Input: part model. Units: mm. Frame: model coordinates. Face numbers are marked on the shaded views. A direction names the side the tool comes from. Coordinates: 2 decimals unless noted, no trailing zeros. Write each loop counter-clockwise with the first axis right and the second up, starting at its lowest first coordinate (ties: lowest second). Pieces come first, ordered by that corner, then holes. Notation, with made-up numbers: (14, -9.75) - (60, -9.75) arc R37 ccw to (60, 26.25) - close; hole circle Ø6 at (9.25, 29). An arc over 180 degrees is marked (long way). Use a Markdown table: item, result. Add a question column.
Q1. Section query D-D (z = 0). Return the cut outline in (x, y).
Q2. Section query C-C (y = 0.7). Return the cut outline in (x, z), then the cut area to 3 significant figures.
Q3. Set-up query: the marked faces 5 and 6. Return all of +Z, -Z, +X, -X, +Y, -Y with unobstructed straight access to the full face (end or side cutting, diameter ignored); none if empty.
Q4. Section query A-A (x = -7.5). Return the cut outline in (y, z).
Q5. Section query B-B (x = 7.5). Return the cut outline in (y, z), then the cut area to 3 significant figures.
Q6. Pin query (flat end, axial travel): P1, Ø1.8, axis at y = 2, z = 0.5, coming from the +X side; P2, Ø6, axis at x = 0, z = 0, coming from the +Y side; P3, Ø1.6, axis at x = 7.5, z = -7.5, coming from the +Y side. Return the tip coordinate at first contact, or that it passes through.
Q7. Mould query, pull axis Y, two halves, no side actions, for the marked faces 1, 2, 3 and 4. Classes: released by +Y, released by -Y, zero draft, split by the parting line, or undercut.
Q8. Material intervals for probe 1 along X at (y, z) = (3, -7.5); probe 2 along X at (y, z) = (3.05, 7.5); probe 3 along Z at (x, y) = (3.5, 3.55), sorted ascending. Write a range as from..to.
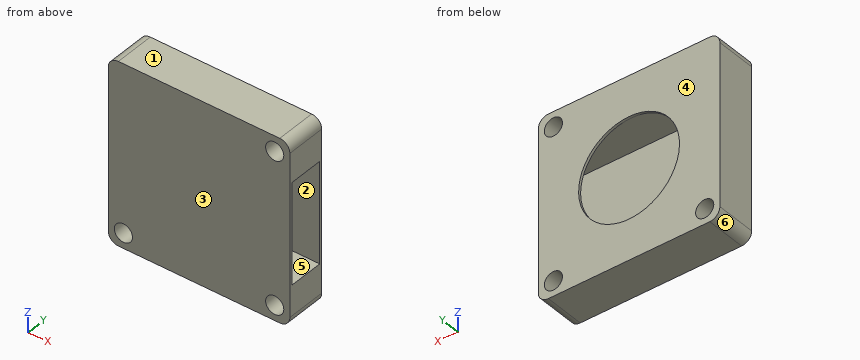
from build123d import *

# Parameters (mm, degrees)
BOSS_EXTRUDE1_DEPTH = 4
CUT_EXTRUDE1_REACH  = 15.342
SKETCH4_R           = 0.9
SKETCH5_R           = 5
CUT_EXTRUDE2_DEPTH  = 3.75
SKETCH6_W           = 10
SKETCH6_H           = 3.5
CUT_EXTRUDE3_DEPTH  = 17.5


with BuildPart() as part:
    # Sketch3 → Boss-Extrude1 (new body)
    with BuildSketch(Plane(origin=(0, 0, 0), x_dir=(1, 0, 0), z_dir=(0, 1, 0))):
        with BuildLine():
            Line((-8, -9), (8, -9))
            ThreePointArc((8, -9), (8.707106781, -8.707106781), (9, -8))
            Line((9, -8), (9, 8))
            ThreePointArc((9, 8), (8.707106781, 8.707106781), (8, 9))
            Line((8, 9), (-8, 9))
            ThreePointArc((-8, 9), (-8.707106781, 8.707106781), (-9, 8))
            Line((-9, 8), (-9, -8))
            ThreePointArc((-9, -8), (-8.707106781, -8.707106781), (-8, -9))
        make_face()
    extrude(amount=BOSS_EXTRUDE1_DEPTH)

    # Sketch4 → Cut-Extrude1 (cut, up to next)
    with BuildSketch(Plane(origin=(0, 4, 0), x_dir=(1, 0, 0), z_dir=(0, 1, 0)), mode=Mode.PRIVATE) as cut_extrude1_sk1:
        with Locations(Location((7.5, -7.5, 0), (0, 0, 270))):
            Circle(SKETCH4_R)
    cut_extrude1_tool1 = extrude(cut_extrude1_sk1.sketch, amount=-CUT_EXTRUDE1_REACH, mode=Mode.PRIVATE) & part.part
    # Sketch4 → Cut-Extrude1 (cut, up to next)
    with BuildSketch(Plane(origin=(0, 4, 0), x_dir=(1, 0, 0), z_dir=(0, 1, 0)), mode=Mode.PRIVATE) as cut_extrude1_sk2:
        with Locations(Location((7.5, 7.5, 0), (0, 0, 270))):
            Circle(SKETCH4_R)
    cut_extrude1_tool2 = extrude(cut_extrude1_sk2.sketch, amount=-CUT_EXTRUDE1_REACH, mode=Mode.PRIVATE) & part.part
    # Sketch4 → Cut-Extrude1 (cut, up to next)
    with BuildSketch(Plane(origin=(0, 4, 0), x_dir=(1, 0, 0), z_dir=(0, 1, 0)), mode=Mode.PRIVATE) as cut_extrude1_sk3:
        with Locations(Location((-7.5, 7.5, 0), (0, 0, 270))):
            Circle(SKETCH4_R)
    cut_extrude1_tool3 = extrude(cut_extrude1_sk3.sketch, amount=-CUT_EXTRUDE1_REACH, mode=Mode.PRIVATE) & part.part
    add(cut_extrude1_tool1.solids().sort_by_distance((7.5, 4, 7.5))[0], mode=Mode.SUBTRACT)
    add(cut_extrude1_tool2.solids().sort_by_distance((7.5, 4, -7.5))[0], mode=Mode.SUBTRACT)
    add(cut_extrude1_tool3.solids().sort_by_distance((-7.5, 4, -7.5))[0], mode=Mode.SUBTRACT)

    # Sketch5 → Cut-Extrude2 (cut)
    with BuildSketch(Plane(origin=(0, 4, 0), x_dir=(1, 0, 0), z_dir=(0, 1, 0))):
        with Locations(Location((0, 0, 0), (0, 0, 270))):
            Circle(SKETCH5_R)
    extrude(amount=-CUT_EXTRUDE2_DEPTH, mode=Mode.SUBTRACT)

    # Sketch6 → Cut-Extrude3 (cut)
    with BuildSketch(Plane(origin=(9, 0, 0), x_dir=(0, 0, -1), z_dir=(1, 0, 0))):
        with Locations((0, 2)):
            Rectangle(SKETCH6_W, SKETCH6_H)
    extrude(amount=-CUT_EXTRUDE3_DEPTH, mode=Mode.SUBTRACT)


solid = part.part
Values follow:
| question | item | result |
|---|---|---|
| 1 | outline | (-9, 0) - (9, 0) - (9, 0.25) - (-8.5, 0.25) - (-8.5, 3.75) - (-5, 3.75) - (-5, 4) - (-9, 4) - close; (5, 3.75) - (9, 3.75) - (9, 4) - (5, 4) - close |
| 2 | outline | (-9, -8) arc R1 ccw to (-8, -9) - (8, -9) arc R1 ccw to (9, -8) - (9, -5) - (-8.5, -5) - (-8.5, 5) - (9, 5) - (9, 8) arc R1 ccw to (8, 9) - (-8, 9) arc R1 ccw to (-9, 8) - close; hole circle Ø1.8 at (-7.5, -7.5); hole circle Ø1.8 at (7.5, -7.5); hole circle Ø1.8 at (7.5, 7.5) |
| 2 | area | 141 mm2 |
| 3 | face 5 | +X |
| 3 | face 6 | -Z, -X, +Y, -Y |
| 4 | outline | (0, -9) - (4, -9) - (4, -8.4) - (0, -8.4) - close; (0, -6.6) - (4, -6.6) - (4, 9) - (0, 9) - close; hole (0.25, -5) - (3.75, -5) - (3.75, 5) - (0.25, 5) - close |
| 5 | outline | (0, -9) - (4, -9) - (4, -8.4) - (0, -8.4) - close; (0, -6.6) - (4, -6.6) - (4, 6.6) - (0, 6.6) - close; (0, 8.4) - (4, 8.4) - (4, 9) - (0, 9) - close; hole (0.25, -5) - (3.75, -5) - (3.75, 5) - (0.25, 5) - close |
| 5 | area | 22.6 mm2 |
| 6 | P1 | x = -8.5 |
| 6 | P2 | y = 0.25 |
| 6 | P3 | through |
| 7 | face 1 | zero draft |
| 7 | face 2 | undercut |
| 7 | face 3 | released by -Y |
| 7 | face 4 | released by +Y |
| 8 | probe 1 | -9..-8.4, -6.6..6.6, 8.4..9 |
| 8 | probe 2 | -9..6.6, 8.4..9 |
| 8 | probe 3 | -9..-5, 5..9 |
